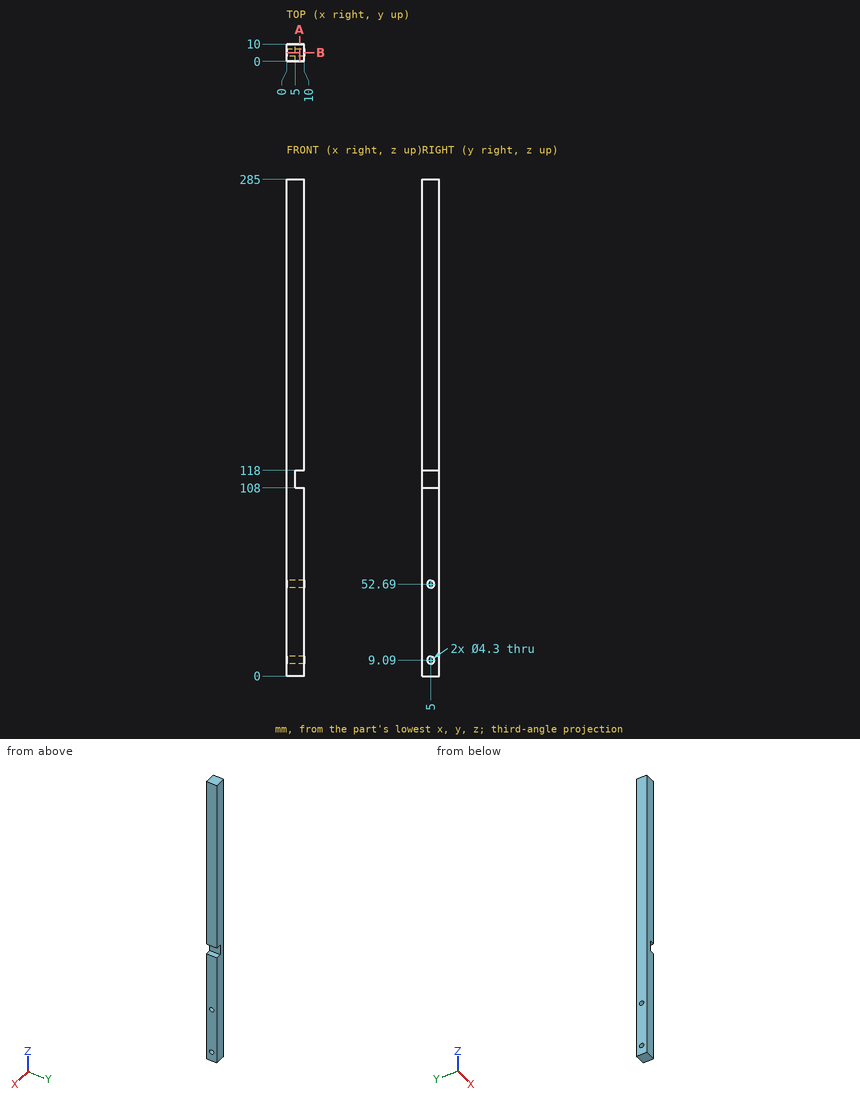
The drawing under review shows one solid part. Ordinate dimensions are in mm from its lowest x, y, z. Round coordinates to 2 decimals unless told otherwise and drop trailing zeros. Write each loop counter-clockwise with the first axis right and the second up, starting at its lowest first coordinate (ties: lowest second). Pieces come first, ordered by that corner, then holes.
(1) Insertion check: pin 1 (6 mm diameter, centred on x = 7, z = 167.5, fed in from -Y); pin 2 (5 mm diameter, centred on y = 3.5, z = 115, fed in from +X). Each pin has a flat end and moves straight along its axis. Give the tip position at first contact, or say it passes through.
(2) We need section A-A on x = 7.5. Give the boundary of the cut face in (y, z).
(3) We need section B-B on y = 5. Give the boundary of the cut face in (x, z).
(4) Wall thickness on L1, parallel to Z at x = 6.25, y = 5; L2, parallel to Z at x = 4.5, y = 5; L3, parallel to Z at x = 5.25, y = 8: over which ranges is each line inside the solid? List them lowest first.
Findings below:
1. pin 1: stops at y = 0
1. pin 2: stops at x = 5
2. outline: (0, 0) - (10, 0) - (10, 108) - (0, 108) - close; (0, 118) - (10, 118) - (10, 285) - (0, 285) - close; hole circle Ø4.3 at (5, 9.09); hole circle Ø4.3 at (5, 52.69)
3. outline: (0, 0) - (10, 0) - (10, 6.94) - (0, 6.94) - close; (0, 11.24) - (10, 11.24) - (10, 50.54) - (0, 50.54) - close; (0, 54.84) - (10, 54.84) - (10, 108) - (5, 108) - (5, 118) - (10, 118) - (10, 285) - (0, 285) - close
4. L1: z = 0 to 6.94, 11.24 to 50.54, 54.84 to 108, 118 to 285
4. L2: z = 0 to 6.94, 11.24 to 50.54, 54.84 to 285
4. L3: z = 0 to 108, 118 to 285
